Autodesk Inventor part; units mm, degrees
ref_plane "XZ Plane" through (0, 0, 0) normal (0, 1, 0) x (-1, 0, 0)
ref_plane "XY Plane" through (0, 0, 0) normal (0, 0, 1) x (1, 0, 0)
sketch "Sketch1" plane through (0, 0, 0) normal (0, 0, 1) x (1, 0, 0)
  line L0 (-5, 6.245) -> (-5, -6.245)
  arc A0 (-5, -6.245) -> (-5, 6.245) centre (0, 0) ccw
  circle A1 centre (0, 0) radius 15
  dimension "d0" = 30
extrude "Extrusion1" add sketch "Sketch1" against normal blind 20
sketch "Sketch2" plane through (0, 0, 0) normal (0, 0, 1) x (1, 0, 0)
  circle A0 centre (0, 0) radius 15
extrude "Extrusion2" add sketch "Sketch2" along normal blind 15
sketch "Sketch3" plane through (0, 0, 15) normal (0, 0, 1) x (1, 0, 0)
  line L0 (-3.175, -2.433) -> (-3.175, 2.433)
  arc A0 (-3.175, -2.433) -> (-3.175, 2.433) centre (0, 0) ccw
  circle A1 centre (0, 0) radius 15
extrude "Extrusion3" add sketch "Sketch3" along normal blind 20
ref_plane "Work Plane1" through (-30.75, 0, 0) normal (1, 0, 0) x (0, 1, 0)
sketch "Sketch4" plane through (-30.75, 0, 0) normal (1, 0, 0) x (0, 1, 0)
  line L0 (15, 35) -> (-15, 35)
  line L1 (-15, -20) -> (15, -20)
  line L2 (-15, 35) -> (-15, -20)
  line L3 (15, 35) -> (15, -20)
  circle A0 centre (0, -10) radius 3
  circle A1 centre (0, 20) radius 2
  point P0 (0, 0)
  dimension "d8" = 4
  dimension "d9" = 6
  dimension "d10" = 10
  dimension "d11" = 15
extrude "Extrusion4" cut sketch "Sketch4" along normal up to surface (30.75 mm away) contours A0 | A1
thread "Thread1"
thread "Thread2"
properties part number "ballscrew coupler" material "Steel, Mild"
Input: part model. Units: mm. Frame: model coordinates. A direction names the side the tool comes from. Round coordinates to 2 decimals unless told otherwise and drop trailing zeros. Write each loop counter-clockwise with the first axis right and the second up, starting at its lowest first coordinate (ties: lowest second). Pieces come first, ordered by that corner, then holes.
1) Ray query, L1, parallel to Y at x = 0, z = 27; L2, parallel to Y at x = 0, z = -6.5; L3, parallel to Z at x = -3, y = 4.5. Return the intervals inside material, ascending.
2) Cut plane B-B (x = -11). Return the cut outline in (y, z).
3) Contact query for flat-ended pins moving along their axis: P1, Ø14.5, axis at x = 0, y = 0, coming from the -Z side; P2, Ø5, axis at x = 10.5, z = 6, coming from the +Y side; P3, Ø2, axis at x = 1.5, y = 1, coming from the +Z side; P4, Ø1.5, axis at x = -3, y = -2, coming from the -Z side. Output: stop coordinate, or through.
4) Draft query along Y for faces 1 (the flat face through (-5, 3, -8)), 2 (the flat face through (-7, 0, -20)), 3 (the cylindrical face through (13.856, 5.745, 7.115)). Return one class per face: pulls with the +Y half, pulls with the -Y half, needs draft (parallel to the pull), parting line crosses it, or undercut.
5) Cut plane A-A (y = 0). Return the cut outline in (x, z) (3 decimals), then the cut area to 3 significant figures.
6) Cut plane C-C (z = 17). Return the cut outline in (x, y) (3 decimals).
7) Cut plane D-D (x = 0). Return the cut outline in (y, z).
8) Reachability of faces 4 (the flat face through (-4, 0, 35)), 5 (the cylindrical face through (8, 0, -10)), 6 (the flat face through (0, 0, 15)), 7 (the cylindrical face through (-9, 0, 18)) from +Z, -Z, +X, -X, +Y, -Y: full face, straight path, thin tool, end or side. Return the list, or none.
Geometry says:
1. L1: y = -15 to -4, 4 to 15
1. L2: y = -15 to -8, 8 to 15
1. L3: z = 0 to 35
2. outline: (-10.2, -20) - (10.2, -20) - (10.2, 35) - (-10.2, 35) - close; hole circle Ø6 at (0, -10); hole circle Ø4 at (0, 20)
3. P1: stops at z = -20
3. P2: stops at y = 12.69
3. P3: stops at z = 15
3. P4: stops at z = 0
4. face 1: undercut
4. face 2: needs draft
4. face 3: parting line crosses it
5. outline: (-15, -20) - (-5, -20) - (-5, -13) - (-15, -13) - close; (-15, -7) - (-5, -7) - (-5, 0) - (8, 0) - (8, -20) - (15, -20) - (15, 35) - (4, 35) - (4, 15) - (-3.175, 15) - (-3.175, 18) - (-15, 18) - close; (-15, 22) - (-3.175, 22) - (-3.175, 35) - (-15, 35) - close
5. area: 1,140 mm2
6. outline: circle Ø30 at (0, 0); hole (-3.175, -2.433) arc R4 ccw (long way) to (-3.175, 2.433) - close
7. outline: (-15, -20) - (-8, -20) - (-8, 0) - (8, 0) - (8, -20) - (15, -20) - (15, 35) - (4, 35) - (4, 15) - (-4, 15) - (-4, 35) - (-15, 35) - close
8. face 4: +Z, +X, -X, +Y, -Y
8. face 5: -Z
8. face 6: +Z
8. face 7: -X
